Part model, mm, in its own coordinate system. A direction names the side the tool comes from. Give positions to 0.01 mm unless a question says otherwise; leave off trailing zeros. Order: outer loops, then holes, each group sorted by start corner. A loop starts at its lowest first (then second) coordinate and runs counter-clockwise, first axis right, second up. Notation, with made-up numbers: (-22.75, -12.75) - (15.25, -12.75) arc R17 ccw to (15.25, 3.25) - close; hole circle Ø11 at (46.5, 31). An arc over 180 degrees is marked (long way). One line per item, written item: value.
```python
from build123d import *

# Parameters (mm, degrees)
SKETCH1_W                = 57.3
SKETCH1_H                = 20.1
BOSS_EXTRUDE1_DEPTH      = 10
SKETCH2_W                = 3
SKETCH2_H                = 8
SKETCH2_W_2              = 6
BOSS_EXTRUDE2_DEPTH      = 20
SKETCH3_R                = 2.5
SKETCH3_R_2              = 1.75
BOSS_EXTRUDE3_DEPTH      = 4
BOSS_EXTRUDE4_START      = -9
SKETCH3_3_R              = 2.5
SKETCH3_3_R_2            = 1.75
BOSS_EXTRUDE4_DEPTH      = 8
CUT_EXTRUDE1_DEPTH       = 53.304158534
CUT_EXTRUDE1_DEPTH_BACK  = 53.304158534
SKETCH3_4_R              = 1.75
CUT_EXTRUDE2_DEPTH       = 35.503001319
CUT_EXTRUDE2_DEPTH_BACK  = 35.503001319
SKETCH4_R                = 1.75
CUT_EXTRUDE3_DEPTH       = 44.832232432
CUT_EXTRUDE3_DEPTH_BACK  = 44.832232432
SKETCH6_R                = 1.75
SKETCH6_R_2              = 6
SKETCH7_R                = 2.5
CUT_EXTRUDE4_DEPTH       = 10
BOSS_EXTRUDE6_DEPTH      = 15.65
BOSS_EXTRUDE6_DEPTH_BACK = 41.65
SKETCH5_R                = 6.5


with BuildPart() as part:
    # Sketch1 → Boss-Extrude1 (new body)
    with BuildSketch(Plane.XY):
        Rectangle(SKETCH1_W, SKETCH1_H)
    extrude(amount=-BOSS_EXTRUDE1_DEPTH)

    # Sketch2 → Boss-Extrude2 (add)
    with BuildSketch(Plane(origin=(0, 0, -10), x_dir=(-1, 0, 0), z_dir=(0, 0, -1))):
        with Locations((-11.5, 0)):
            Rectangle(SKETCH2_W, SKETCH2_H)
        Rectangle(SKETCH2_W_2, SKETCH2_H)
        with Locations((11.5, 0)):
            Rectangle(SKETCH2_W, SKETCH2_H)
    extrude(amount=BOSS_EXTRUDE2_DEPTH)

    # Sketch3 → Boss-Extrude3 (add)
    with BuildSketch(Plane(origin=(13, 0, 0), x_dir=(0, 0, -1), z_dir=(1, 0, 0))):
        with Locations((22.39, 0)):
            Circle(SKETCH3_R)
        with Locations((22.39, 0)):
            Circle(SKETCH3_R_2, mode=Mode.SUBTRACT)
    boss_extrude3 = extrude(amount=-BOSS_EXTRUDE3_DEPTH)

    # Sketch3<3> → Boss-Extrude4 (add)
    with BuildSketch(Plane(origin=(13, 0, 0), x_dir=(0, 0, -1), z_dir=(1, 0, 0)).offset(BOSS_EXTRUDE4_START)):
        with Locations((22.39, 0)):
            Circle(SKETCH3_3_R)
        with Locations((22.39, 0)):
            Circle(SKETCH3_3_R_2, mode=Mode.SUBTRACT)
    extrude(amount=-BOSS_EXTRUDE4_DEPTH)

    # Mirror1: Boss-Extrude3 across plane
    add(boss_extrude3.mirror(Plane(origin=(0, 0, 0), x_dir=(0, 0, 1), z_dir=(1, 0, 0))))

    # Sketch3<4> → Cut-Extrude1 (cut, two sides: drawn at the far end of the back side and taken through both)
    with BuildSketch(Plane(origin=(13, 0, 0), x_dir=(0, 0, -1), z_dir=(1, 0, 0)).offset(-CUT_EXTRUDE1_DEPTH_BACK)):
        with Locations((22.39, 0)):
            Circle(SKETCH3_4_R)
        with BuildLine():
            Line((30, 4), (22.39, 4))
            ThreePointArc((22.39, 4), (25.218427125, 2.828427125), (26.39, 0))
            ThreePointArc((26.39, 0), (25.218427125, -2.828427125), (22.39, -4))
            Line((22.39, -4), (30, -4))
            Line((30, -4), (30, 4))
        make_face()
    extrude(amount=CUT_EXTRUDE1_DEPTH + CUT_EXTRUDE1_DEPTH_BACK, mode=Mode.SUBTRACT)

    # Sketch4 → Cut-Extrude2 (cut, two sides: drawn at the far end of the back side and taken through both)
    with BuildSketch(Plane(origin=(0, 0, -10), x_dir=(-1, 0, 0), z_dir=(0, 0, -1)).offset(-CUT_EXTRUDE2_DEPTH_BACK)):
        with Locations((-21.65, 0)):
            Circle(SKETCH4_R)
        with Locations((21.65, 0)):
            Circle(SKETCH4_R)
    extrude(amount=CUT_EXTRUDE2_DEPTH + CUT_EXTRUDE2_DEPTH_BACK, mode=Mode.SUBTRACT)

    # Sketch6 → Cut-Extrude3 (cut, two sides: drawn at the far end of the back side and taken through both)
    with BuildSketch(Plane(origin=(0, 10.05, 0), x_dir=(1, 0, 0), z_dir=(0, 1, 0)).offset(-CUT_EXTRUDE3_DEPTH_BACK)):
        with Locations(Location((-12, 6, 0), (0, 0, 270))):
            Circle(SKETCH6_R)
        with Locations(Location((12, 6, 0), (0, 0, 270))):
            Circle(SKETCH6_R)
        with Locations((0, 1.75)):
            Circle(SKETCH6_R_2)
    extrude(amount=CUT_EXTRUDE3_DEPTH + CUT_EXTRUDE3_DEPTH_BACK, mode=Mode.SUBTRACT)

    # Sketch7 → Cut-Extrude4 (cut)
    with BuildSketch(Plane(origin=(28.65, 0, 0), x_dir=(0, 0, -1), z_dir=(1, 0, 0))):
        with Locations((5, 5.05)):
            Circle(SKETCH7_R)
    cut_extrude4 = extrude(amount=-CUT_EXTRUDE4_DEPTH, mode=Mode.SUBTRACT)

    # Mirror2: Cut-Extrude4 across plane
    add(cut_extrude4.mirror(Plane(origin=(0, 0, 0), x_dir=(0, 0, 1), z_dir=(1, 0, 0))), mode=Mode.SUBTRACT)

    # Sketch5 → Boss-Extrude6 (add, two sides: drawn at the far end of the back side and taken through both)
    with BuildSketch(Plane(origin=(13, 0, 0), x_dir=(0, 0, -1), z_dir=(1, 0, 0)).offset(-BOSS_EXTRUDE6_DEPTH_BACK)):
        with Locations((22.39, 0)):
            Circle(SKETCH5_R)
    extrude(amount=BOSS_EXTRUDE6_DEPTH + BOSS_EXTRUDE6_DEPTH_BACK)


solid = part.part
```
1) Slice it at D-D on z = -13. Write the cut outline in (x, y), then the cut area to 3 significant figures.
Answer:
outline: (-13, -4) - (-10, -4) - (-10, 4) - (-13, 4) - close; (-3, -4) - (3, -4) - (3, 4) - (-3, 4) - close; (10, -4) - (13, -4) - (13, 4) - (10, 4) - close
area: 96.0 mm2
2) Slice it at A-A on x = -21.65. Write the cut outline in (y, z), then the cut area to 3 significant figures.
Answer:
outline: (-10.05, -10) - (-1.75, -10) - (-1.75, 0) - (-10.05, 0) - close; circle Ø13 at (0, -22.39); (1.75, -10) - (10.05, -10) - (10.05, 0) - (1.75, 0) - close; hole circle Ø5 at (5.05, -5)
area: 279 mm2
3) Two-plate mould, pull along Z, no slides. Class faces 1 (the face through (28.65, 0, -5)), 2 (the face through (13.735, -0.141, -6.228)), 3 (the face through (-17, 0, 0)): pulls with the +Z half, pulls with the -Z half, needs draft (parallel to the pull), parting line crosses it, or undercut.
Answer:
face 1: needs draft
face 2: undercut
face 3: pulls with the +Z half
4) Which spindle directions (+Z, -Z, +X, -X, +Y, -Y) get a long thin tool onto all of the face, cutting with end or side? Do faces 4 (the face through (18.65, 5, -5)), 5 (the face through (-23.72, 5.801, -7.385)), 6 (the face through (-11, -4, -14)), 7 (the face through (-11, 4, -14)). Say none if no direction does.
Answer:
face 4: +X
face 5: -X
face 6: +X, -X, -Y
face 7: +X, -X, +Y
5) Wall check: line 1 along X through (y, z) = (-4.5, -1.75); line 2 along X through (y, z) = (0, -5); line 3 along Z through (x, y) = (12, 1.75). Give the ranges that are in metal, low to high. Write a range as [from, to].
Answer:
line 1: x = [-28.65, -6], [6, 28.65]
line 2: x = [-28.65, -23.4], [-19.9, -13.44], [-10.56, -5.04], [5.04, 10.56], [13.44, 19.9], [23.4, 28.65]
line 3: z = [-28.65, -7.75], [-4.25, 0]
6) Drop flat-ended pins along their axis: P1, Ø5, axis at x = -11.5, z = -16.5, coming from the -Y side; P2, Ø4, axis at x = -12, z = -6, coming from the +Y side; P3, Ø1.5, axis at y = 6, z = -5.5, coming from the +X side; P4, Ø5, axis at y = 2, z = -13, coming from the +X side. Give the stop position or say it passes through.
Answer:
P1: stops at y = -5.55
P2: stops at y = 10.05
P3: stops at x = 18.65
P4: stops at x = 13
7) Slice it at B-B on z = -1.75. Write the cut outline in (x, y).
Answer:
outline: (-28.65, -10.05) - (-6, -10.05) - (-6, 10.05) - (-28.65, 10.05) - close; (6, -10.05) - (28.65, -10.05) - (28.65, 10.05) - (6, 10.05) - close; hole circle Ø3.5 at (-21.65, 0); hole circle Ø3.5 at (21.65, 0)
8) Slice it at C-C on y = 5.05. Write the cut outline in (x, z).
Answer:
outline: (-28.65, -26.48) - (28.65, -26.48) - (28.65, -18.3) - (-28.65, -18.3) - close; (-28.65, -10) - (28.65, -10) - (28.65, -7.5) - (18.65, -7.5) - (18.65, -2.5) - (28.65, -2.5) - (28.65, 0) - (5.74, 0) arc R6 cw (long way) to (-5.74, 0) - (-28.65, 0) - (-28.65, -2.5) - (-18.65, -2.5) - (-18.65, -7.5) - (-28.65, -7.5) - close; hole circle Ø3.5 at (-12, -6); hole circle Ø3.5 at (12, -6)
